```python
from build123d import *

# Parameters (mm, degrees)
F1_DEPTH = 4
F2_R     = 10
F3_R     = 5


with BuildPart() as f1:
    # F0 (on Front) → F1 (new body)
    with BuildSketch(Plane.XZ):
        Polygon((50, 50), (50, 0), (700, 0), (700, 50), (712.5, 50), (750, 50), (750, 356.37), (712.5, 356.37), (700, 356.37), (700, 406.37), (50, 406.37), (50, 356.37), (37.5, 356.37), (0, 356.37), (0, 50), (37.5, 50), align=None)
        with BuildLine():
            ThreePointArc((40.75, 62.5), (39.798097, 60.201903), (37.5, 59.25))
            ThreePointArc((37.5, 59.25), (35.201903, 64.798097), (40.75, 62.5))
        make_face(mode=Mode.SUBTRACT)
        with BuildLine():
            ThreePointArc((715.75, 62.5), (714.798097, 60.201903), (712.5, 59.25))
            ThreePointArc((712.5, 59.25), (710.201903, 64.798097), (715.75, 62.5))
        make_face(mode=Mode.SUBTRACT)
        with BuildLine():
            ThreePointArc((40.75, 343.87), (35.201903, 341.571903), (37.5, 347.12))
            ThreePointArc((37.5, 347.12), (39.798097, 346.168097), (40.75, 343.87))
        make_face(mode=Mode.SUBTRACT)
        with BuildLine():
            ThreePointArc((715.75, 343.87), (710.201903, 341.571903), (712.5, 347.12))
            ThreePointArc((712.5, 347.12), (714.798097, 346.168097), (715.75, 343.87))
        make_face(mode=Mode.SUBTRACT)
    extrude(amount=F1_DEPTH)

    # F2
    f2_edges = [f1.edges().sort_by_distance(p)[0] for p in [
        (0, -2, 356.37),
        (50, -2, 406.37),
        (0, -2, 50),
        (50, -2, 0),
        (700, -2, 0),
        (750, -2, 50),
        (750, -2, 356.37),
        (700, -2, 406.37),
    ]]
    fillet(f2_edges, radius=F2_R)

    # F3
    f3_edges = [f1.edges().sort_by_distance(p)[0] for p in [
        (700, -2, 356.37),
        (700, -2, 50),
        (50, -2, 50),
        (50, -2, 356.37),
    ]]
    fillet(f3_edges, radius=F3_R)


solid = f1.part
```
Verification items for the finished model (mm, model axes). Round coordinates to 2 decimals unless told otherwise and drop trailing zeros. Loops run counter-clockwise (first coordinate to the right, second up) from the corner with the lowest first, then second, coordinate; pieces in that order, holes last. Notation, with made-up numbers: (66.5, -19.5) -> (77.5, -19.5) arc R21 ccw to (77.5, 1.5) -> close; hole circle Ø9 at (-4, -13). An arc over 180 degrees is marked (long way). Answer as a JSON object with one key per item and string values.
Q1. Scan lines: line 1 (X direction, y = -2.7, z = 62.5); line 2 (Z direction, x = 712.5, y = -2.1); line 3 (X direction, y = -2.8, z = 26.5). Record each from-to range of solid material in increasing order. Write a range as from..to.
Data:
{"line 1": "x = 0..34.25, 40.75..709.25, 715.75..750", "line 2": "z = 50..59.25, 65.75..340.62, 347.12..356.37", "line 3": "x = 50..700"}
Q2. Go/stop test with flat-tipped pins: P1, Ø1.2, axis at y = -1, z = 380, coming from the +X side; P2, Ø6, axis at x = 37.5, z = 62.5, coming from the +Y side; P3, Ø2, axis at y = -2.5, z = 19.5, coming from the -X side. Record where each tip stops, or that it passes through.
Data:
{"P1": "stops at x = 700", "P2": "passes through", "P3": "stops at x = 50"}
Q3. Section check A-A (y = -1.6). Record the boundary of the cut face in (x, z).
Data:
{"outline": "(0, 60) arc R10 ccw to (10, 50) -> (45, 50) arc R5 cw to (50, 45) -> (50, 10) arc R10 ccw to (60, 0) -> (690, 0) arc R10 ccw to (700, 10) -> (700, 45) arc R5 cw to (705, 50) -> (740, 50) arc R10 ccw to (750, 60) -> (750, 346.37) arc R10 ccw to (740, 356.37) -> (705, 356.37) arc R5 cw to (700, 361.37) -> (700, 396.37) arc R10 ccw to (690, 406.37) -> (60, 406.37) arc R10 ccw to (50, 396.37) -> (50, 361.37) arc R5 cw to (45, 356.37) -> (10, 356.37) arc R10 ccw to (0, 346.37) -> close; hole circle Ø6.5 at (37.5, 62.5); hole circle Ø6.5 at (37.5, 343.87); hole circle Ø6.5 at (712.5, 62.5); hole circle Ø6.5 at (712.5, 343.87)"}
